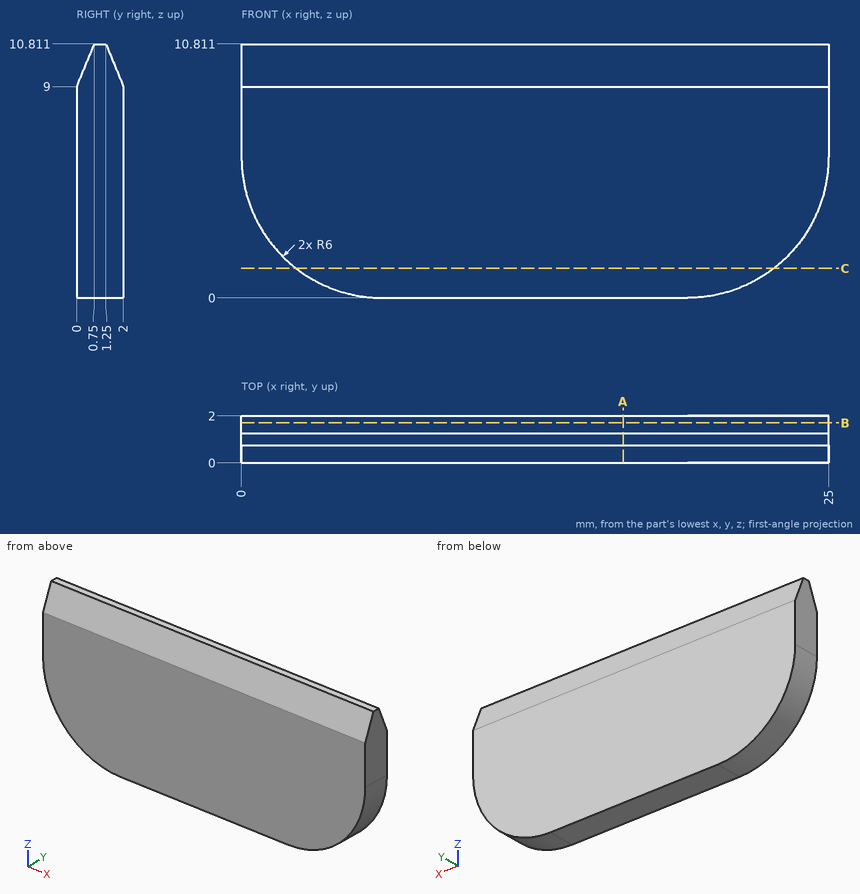
Geometry: see drawing. Coordinates: mm, zero at the bounding-box minimum. Round coordinates to 2 decimals unless told otherwise and drop trailing zeros. Order: outer loops, then holes, each group sorted by start corner. A loop starts at its lowest first (then second) coordinate and runs counter-clockwise, first axis right, second up. Notation, with made-up numbers: (-16.5, 2.25) -> (2.5, 2.25) arc R11 ccw to (2.5, 15.25) -> close; hole circle Ø4 at (63, 31). An arc over 180 degrees is marked (long way). Write each question's results on one line, items separated by ' | '.
Q1. Section query B-B (y = 1.7). Output: boundary loops of the cut face in (x, z).
Response values:
outline: (0, 6) arc R6 ccw to (6, 0) -> (19, 0) arc R6 ccw to (25, 6) -> (25, 9.72) -> (0, 9.72) -> close
Q2. Section query C-C (z = 1.25). Output: boundary loops of the cut face in (x, y).
Response values:
outline: (2.33, 0) -> (22.67, 0) -> (22.67, 2) -> (2.33, 2) -> close
Q3. Ray query, line 1 along X through (y, z) = (0.4, 1.5); line 2 along Z through (x, y) = (12.25, 1.6) (1 decimal); line 3 along Z through (x, y) = (2.5, 0.5) (1 decimal). Return the intervals inside material, ascending.
Response values:
line 1: 2.03 to 22.97 | line 2: 0 to 10 | line 3: 1.1 to 10.2
Q4. Section query A-A (x = 16.25). Output: boundary loops of the cut face in (y, z).
Response values:
outline: (0, 0) -> (2, 0) -> (2, 9) -> (1.25, 10.81) -> (0.75, 10.81) -> (0, 9) -> close
